Autodesk Inventor part; units mm, degrees
ref_plane "YZ Plane" through (0, 0, 0) normal (1, 0, 0) x (0, 1, 0)
ref_plane "XZ Plane" through (0, 0, 0) normal (0, 1, 0) x (-1, 0, 0)
ref_plane "XY Plane" through (0, 0, 0) normal (0, 0, 1) x (1, 0, 0)
sketch "Boceto1" plane through (0, 0, 0) normal (0, 0, 1) x (1, 0, 0)
  line L0 (-12.1173, 0.2988) -> (-22.1173, 0.2988)
  line L1 (-22.1173, 0.2988) -> (-22.1173, -2.2012)
  line L2 (-22.1173, -2.2012) -> (-51.1173, -2.2012)
  line L3 (-51.1173, -2.2012) -> (-51.1173, 0.2988)
  line L4 (-51.1173, 0.2988) -> (-75.1173, 0.2988)
  line L5 (-75.1173, 0.2988) -> (-75.1173, -42.7012)
  line L6 (-75.1173, -42.7012) -> (-12.1173, -42.7012)
  line L7 (-12.1173, -42.7012) -> (-12.1173, 0.2988)
  circle A0 centre (-18.1173, -9.2012) radius 1.75
  circle A1 centre (-67.1173, -9.2012) radius 1.75
  circle A2 centre (-18.1173, -38.2012) radius 1.7568
  circle A3 centre (-27.1173, -27.7012) radius 5
  point P0 (0, 0)
extrude "Extrusión1" add sketch "Boceto1" along normal blind 5
properties part number "carro x lado motor pieza 2parte 2-2"
Read the model definition and answer for the solid it produces. Units are mm, in the model's axes. A direction names the side the tool comes from. Coordinates: 2 decimals unless noted, no trailing zeros. Loops run counter-clockwise (first coordinate to the right, second up) from the corner with the lowest first, then second, coordinate; pieces in that order, holes last.
Q1. The part is cut by section C-C on z = 0.75. Write down the section's boundary in (x, y).
Q2. The part is cut by section B-B on y = -28.5. Write down the section's boundary in (x, z), and give its area (3 significant figures).
Q3. The part is cut by section A-A on y = -10. Write down the section's boundary in (x, z), and give its area (3 significant figures).
Q4. The mould has two halves that part along X. Classify faces 1 (the face through (-12.117, -22, 2)), 2 (the face through (-63, 0.299, 2)), 3 (the face through (-75.117, -21, 2)), 4 (the face through (-18.498, -36.486, 2.465)): +X half, -X half, draft (parallel to the pull), parting line (faces both ways), or undercut.
Q5. Which of the six approach directions +Z, -Z, +X, -X, +Y, -Y give full straight-line access (tool end or side, diameter ignored) to faces 5 (the face through (-36, -2.201, 2)), 6 (the face through (-44, -21, 5))?
Q6. Consider probe 1 along X at (y, z) = (-9, 2.35); probe 2 along X at (y, z) = (-1.5, 0.25); probe 3 along Y at (x, z) = (-49, 4.45). Determine where each line is inside the solid, lowest interval first.
Q7. This flat-tipped pin is pushed along its axis until it touches: pin 1 Ø2 at (x, z) = (-44, 2.5) entering from +Y. Where does it stop, or does it pass through?
Q8. The part is cut by section D-D on x = -67. Write down the section's boundary in (y, z), and give its area (3 significant figures).
Results below:
1. outline: (-75.12, -42.7) - (-12.12, -42.7) - (-12.12, 0.3) - (-22.12, 0.3) - (-22.12, -2.2) - (-51.12, -2.2) - (-51.12, 0.3) - (-75.12, 0.3) - close; hole circle Ø3.5 at (-67.12, -9.2); hole circle Ø10 at (-27.12, -27.7); hole circle Ø3.51 at (-18.12, -38.2); hole circle Ø3.5 at (-18.12, -9.2)
2. outline: (-75.12, 0) - (-32.05, 0) - (-32.05, 5) - (-75.12, 5) - close; (-22.18, 0) - (-12.12, 0) - (-12.12, 5) - (-22.18, 5) - close
2. area: 266 mm2
3. outline: (-75.12, 0) - (-68.67, 0) - (-68.67, 5) - (-75.12, 5) - close; (-65.56, 0) - (-19.67, 0) - (-19.67, 5) - (-65.56, 5) - close; (-16.56, 0) - (-12.12, 0) - (-12.12, 5) - (-16.56, 5) - close
3. area: 284 mm2
4. face 1: +X half
4. face 2: draft
4. face 3: -X half
4. face 4: undercut
5. face 5: +Z, -Z, +Y
5. face 6: +Z, +X, -X, +Y, -Y
6. probe 1: x = -75.12 to -68.86, -65.38 to -19.86, -16.38 to -12.12
6. probe 2: x = -75.12 to -51.12, -22.12 to -12.12
6. probe 3: y = -42.7 to -2.2
7. pin 1: stops at y = -2.2
8. outline: (-42.7, 0) - (-10.95, 0) - (-10.95, 5) - (-42.7, 5) - close; (-7.46, 0) - (0.3, 0) - (0.3, 5) - (-7.46, 5) - close
8. area: 198 mm2
